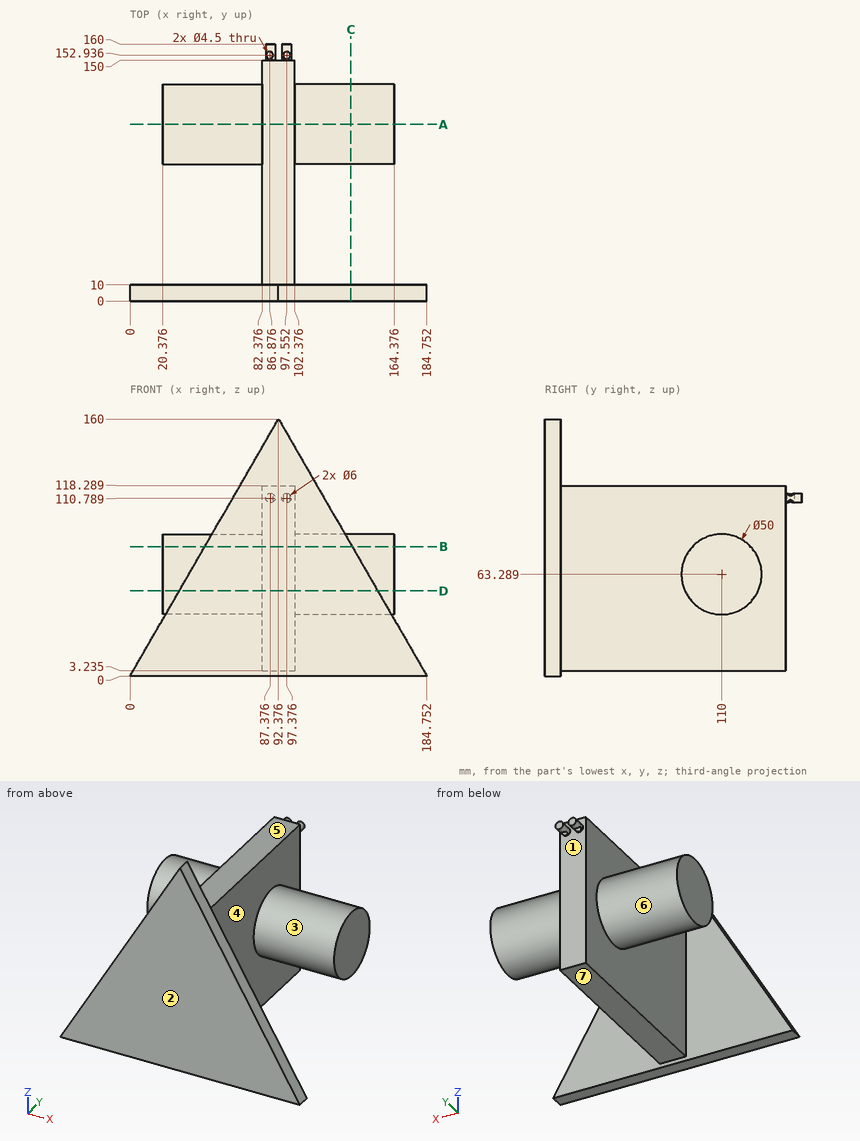
The drawing under review shows one solid part. Ordinate dimensions are in mm from its lowest x, y, z. A direction names the side the tool comes from. Give positions to 0.01 mm unless a question says otherwise; leave off trailing zeros. Write each loop counter-clockwise with the first axis right and the second up, starting at its lowest first coordinate (ties: lowest second). Pieces come first, ordered by that corner, then holes. Notation, with made-up numbers: (69, -0.5) -> (97, -0.5) arc R17 ccw to (97, 11.5) -> close; hole circle Ø3 at (21.5, 42). An arc over 180 degrees is marked (long way). Use CSV: the item, a comma, the result in double quotes.
Q1. Take a section at D-D, the plane z = 53. Write out the cut boundary in (x, y) (1 decimal), then the cut area to 3 significant figures.
Conclusion:
outline,"(20.4, 87.2) -> (82.4, 87.2) -> (82.4, 10) -> (30.6, 10) -> (30.6, 0) -> (154.2, 0) -> (154.2, 10) -> (102.4, 10) -> (102.4, 87.2) -> (164.4, 87.2) -> (164.4, 132.8) -> (102.4, 132.8) -> (102.4, 150) -> (82.4, 150) -> (82.4, 132.8) -> (20.4, 132.8) -> close"
area,"9,690 mm2"
Q2. Tool access review of the marked faces 5, 6 and 7: name each direction out of +Z, -Z, +X, -X, +Y, -Y from which nothing blocks a thin tool from reaching the whole face with its end or side.
Conclusion:
face 5,"+Z, +X, -X, +Y"
face 6,"-X"
face 7,"-Z, +X, -X, +Y"
Q3. Take a section at A-A, the plane y = 110. Write out the cut boundary in (x, z) (1 decimal).
Conclusion:
outline,"(20.4, 38.3) -> (82.4, 38.3) -> (82.4, 3.2) -> (102.4, 3.2) -> (102.4, 38.3) -> (164.4, 38.3) -> (164.4, 88.3) -> (102.4, 88.3) -> (102.4, 118.3) -> (82.4, 118.3) -> (82.4, 88.3) -> (20.4, 88.3) -> close"
Q4. Take a section at C-C, the plane x = 137.5. Write out the cut boundary in (y, z).
Conclusion:
outline,"(0, 0) -> (10, 0) -> (10, 81.84) -> (0, 81.84) -> close; circle Ø50 at (110, 63.29)"
Q5. Take a section at B-B, the plane z = 80.5. Write out the cut boundary in (x, y) (1 decimal).
Conclusion:
outline,"(20.4, 91.9) -> (82.4, 91.9) -> (82.4, 10) -> (46.5, 10) -> (46.5, 0) -> (138.3, 0) -> (138.3, 10) -> (102.4, 10) -> (102.4, 91.9) -> (164.4, 91.9) -> (164.4, 128.1) -> (102.4, 128.1) -> (102.4, 150) -> (82.4, 150) -> (82.4, 128.1) -> (20.4, 128.1) -> close"
Q6. For P1, Ø7, axis at x = 86.88, y = 152.94, coming from the +Z side; P2, Ø8, axis at x = 126.5, y = 114, coming from the +Z side; P3, Ø3, axis at x = 67.5, z = 19, coming from the +Y side, all flat-tipped, find the tip position at first contact; note any pin that passes through.
Conclusion:
P1,"z = 118.29"
P2,"z = 88.29"
P3,"y = 10"
Q7. Mouldability with a two-part tool opening along Y and no side actions: class the marked faces 1, 2, 3 and 4 as pulls with the +Y half, pulls with the -Y half, needs draft (parallel to the pull), parting line crosses it, or undercut.
Conclusion:
face 1,"pulls with the +Y half"
face 2,"pulls with the -Y half"
face 3,"undercut"
face 4,"undercut"
Q8. To check wall thickness, follow probe 1 along X at (y, z) = (21, 98.5); probe 2 along X at (y, z) = (91, 59.5); probe 3 along Y at (x, z) = (63.5, 25). State the ranges of each line that lie inside material, in increasing order. Write a range as [from, to].
Conclusion:
probe 1,"[82.38, 102.38]"
probe 2,"[20.38, 164.38]"
probe 3,"[0, 10]"
